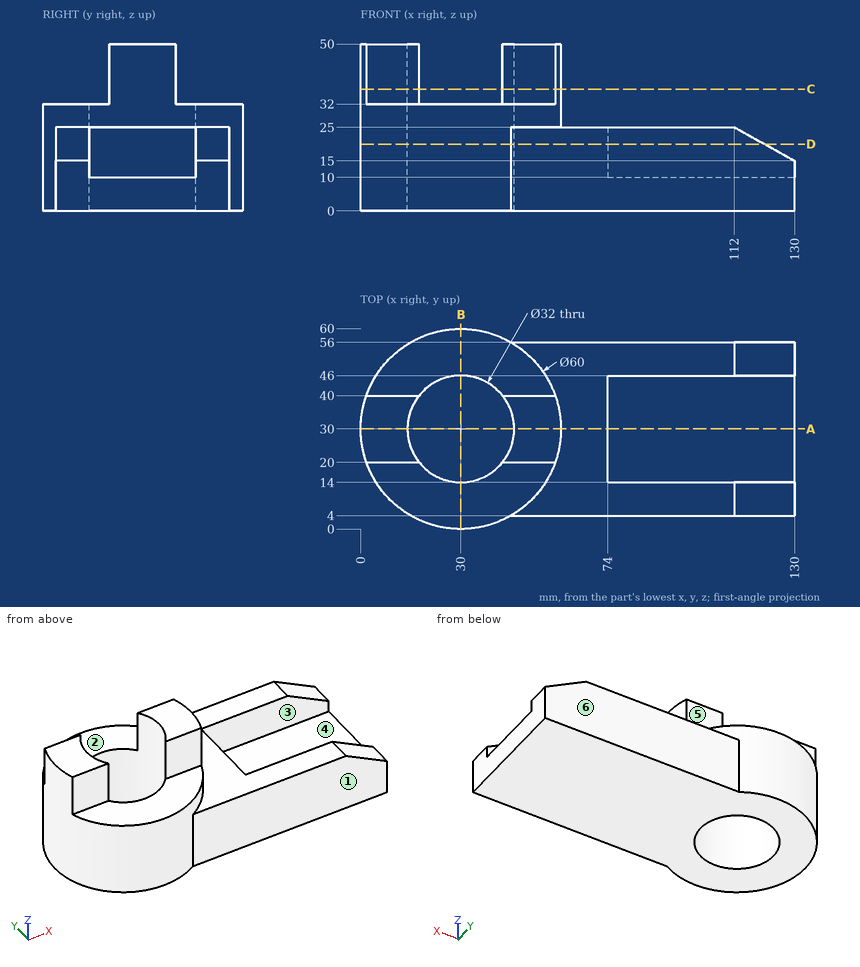
Drawing for the job (mm, zero at the part's lowest x, y, z). A direction names the side the tool comes from. Give positions to 0.01 mm unless a question says otherwise; leave off trailing zeros. Loops run counter-clockwise (first coordinate to the right, second up) from the corner with the lowest first, then second, coordinate; pieces in that order, holes last. Notation, with made-up numbers: M 42,76 L 65,76 A29 cw 65,106 Z; hole C 82.5,0 d2. An arc over 180 degrees is marked long. One line per question, with ' | ' between items. Start each with the question number.
1. Saw through at C-C on z = 36.5. Give the cut face in (x, y).
2. Two-plate mould, pull along Y, no slides. Class the marked faces 1, 2 and 3: pulls with the +Y half, pulls with the -Y half, needs draft (parallel to the pull), parting line crosses it, or undercut.
3. Saw through at D-D on z = 20. Give the cut face in (x, y), plus the area to 3 significant figures.
4. Saw through at B-B on x = 30. Give the cut face in (y, z), plus the area to 3 significant figures.
5. Probe L1, parallel to X at y = 30, z = 39; L2, parallel to X at y = 30, z = 13. List the from-to ranges inside material, lowest first. Write a range as from..to.
6. Flat gauge pins, fed straight in: pin 1 (4.5 mm diameter, centred on x = 50, z = 39, fed in from -Y); pin 2 (12 mm diameter, centred on x = 109, z = 17, fed in from +Y); pin 3 (12 mm diameter, centred on y = 23.5, z = 15, fed in from +X); pin 4 (15.5 mm diameter, centred on x = 71.5, y = 30, fed in from +Z). Where does each tip first touch, or does it go through?
7. Saw through at A-A on y = 30. Give the cut face in (x, z), plus the area to 3 significant figures.
8. 3-axis set-ups, long thin cutter, end or side, ignore diameter. For the marked faces 4, 5 and 6: which of +Z, -Z, +X, -X, +Y, -Y reach the whole face in a straight line?
Result sheet:
1) outline: M 1.72,20 L 17.51,20 A16 cw 17.51,40 L 1.72,40 A30 ccw Z; M 42.49,20 L 58.28,20 A30 ccw 58.28,40 L 42.49,40 A16 cw Z
2) face 1: pulls with the -Y half | face 2: needs draft | face 3: undercut
3) outline: M 44.97,4 L 121,4 L 121,14 L 74,14 L 74,46 L 121,46 L 121,56 L 44.97,56 A30 ccw long Z; hole C 30,30 d32 | area: 3,920 mm^2
4) outline: M 0,0 L 14,0 L 14,32 L 0,32 Z; M 46,0 L 60,0 L 60,32 L 46,32 Z | area: 896 mm^2
5) L1: x = 0..14, 46..60 | L2: x = 0..14, 46..74
6) pin 1: stops at y = 20 | pin 2: stops at y = 56 | pin 3: stops at x = 130 | pin 4: stops at z = 25
7) outline: M 0,0 L 14,0 L 14,50 L 0,50 Z; M 46,0 L 130,0 L 130,10 L 74,10 L 74,25 L 60,25 L 60,50 L 46,50 Z | area: 2,310 mm^2
8) face 4: +Z, +X | face 5: +Z, +X, -X, +Y | face 6: +Z, -Z, +X, +Y
